Model file for the job. Use its own axes, mm. Coordinates: 2 decimals unless noted, no trailing zeros. Loops run counter-clockwise (first coordinate to the right, second up) from the corner with the lowest first, then second, coordinate; pieces in that order, holes last. Notation, with made-up numbers: (49, -28.5) -> (107, -28.5) arc R22 ccw to (107, -0.5) -> close; hole circle Ø4 at (-24.5, 77). An arc over 180 degrees is marked (long way). Use one line per item in the form item = value.
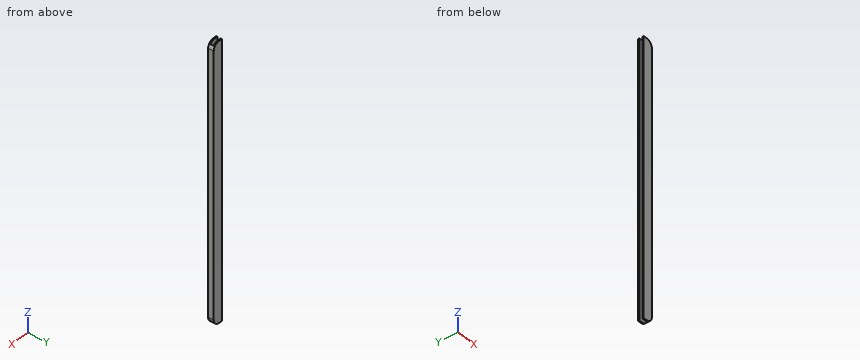
```python
from build123d import *

# Parameters (mm, degrees)
SKETCH2_W           = 15
SKETCH2_H           = 432
BOSS_EXTRUDE1_DEPTH = 9
SKETCH3_W           = 432
SKETCH3_H           = 5
CUT_EXTRUDE1_DEPTH  = 13
FILLET1_R           = 10
FILLET2_R           = 10


with BuildPart() as part:
    # Sketch2 → Boss-Extrude1 (new body)
    with BuildSketch(Plane(origin=(0, 0, 0), x_dir=(1, 0, 0), z_dir=(0, 1, 0))):
        with Locations((-75.63559322, -170.618644068)):
            Rectangle(SKETCH2_W, SKETCH2_H)
    extrude(amount=BOSS_EXTRUDE1_DEPTH)

    # Sketch3 → Cut-Extrude1 (cut)
    with BuildSketch(Plane.ZY.offset(83.13559322)):
        with Locations((170.618644068, 4.5)):
            Rectangle(SKETCH3_W, SKETCH3_H)
    extrude(amount=-CUT_EXTRUDE1_DEPTH, mode=Mode.SUBTRACT)

    # Fillet1
    # the kernel refuses this fillet: 10 mm, written as the material it takes off along each edge
    with BuildSketch(Plane(origin=(-68.13559322, -25, 386.618644068), x_dir=(0, 0, -1), z_dir=(0, 1, 0))) as fillet1_piece_1:
        with BuildLine():
            CenterArc((FILLET1_R, FILLET1_R), FILLET1_R, 180, 90)
            Line((0, FILLET1_R), (0, 0))
            Line((0, 0), (FILLET1_R, 0))
        make_face()
    extrude(amount=59, mode=Mode.SUBTRACT)

    # Fillet2
    # the kernel refuses this fillet: 10 mm, written as the material it takes off along each edge
    with BuildSketch(Plane(origin=(-68.13559322, -25, -45.381355932), x_dir=(-1, 0, 0), z_dir=(0, 1, 0))) as fillet2_piece_1:
        with BuildLine():
            CenterArc((FILLET2_R, FILLET2_R), FILLET2_R, 180, 90)
            Line((0, FILLET2_R), (0, 0))
            Line((0, 0), (FILLET2_R, 0))
        make_face()
    extrude(amount=59, mode=Mode.SUBTRACT)


solid = part.part
```
Q1. Band-saw the part on A-A, the plane z = 132. Write the cut outline in (x, y).
Result:
outline = (-83.14, 0) -> (-68.14, 0) -> (-68.14, 9) -> (-83.14, 9) -> (-83.14, 7) -> (-70.14, 7) -> (-70.14, 2) -> (-83.14, 2) -> close
Q2. Band-saw the part on C-C, the plane y = 4. Write the cut outline in (x, z).
Result:
outline = (-70.14, -41.38) arc R10 ccw to (-68.14, -35.38) -> (-68.14, 376.62) arc R10 ccw to (-70.14, 382.62) -> close
Q3. Wall check: line 1 along Y through (x, z) = (-79.5, 113); line 2 along Z through (x, y) = (-78, 0.5); line 3 along X through (y, z) = (6.5, 137). Give the ranges that are in metal, low to high.
Result:
line_1 = 0 to 2, 7 to 9
line_2 = -45.38 to 386.62
line_3 = -70.14 to -68.14
Q4. Pin check, flat tip, straight feed: pin 1 Ø1.5 at (y, z) = (3.5, 90.5) entering from -X. Stop position of the tip, or through.
Result:
pin_1 = -70.14
Q5. Band-saw the part on B-B, the plane x = -73. Write the cut outline in (y, z), and give its area (3 significant figures).
Result:
outline = (0, -43.96) -> (2, -43.96) -> (2, 385.2) -> (0, 385.2) -> close; (7, -43.96) -> (9, -43.96) -> (9, 385.2) -> (7, 385.2) -> close
area = 1,720 mm2
